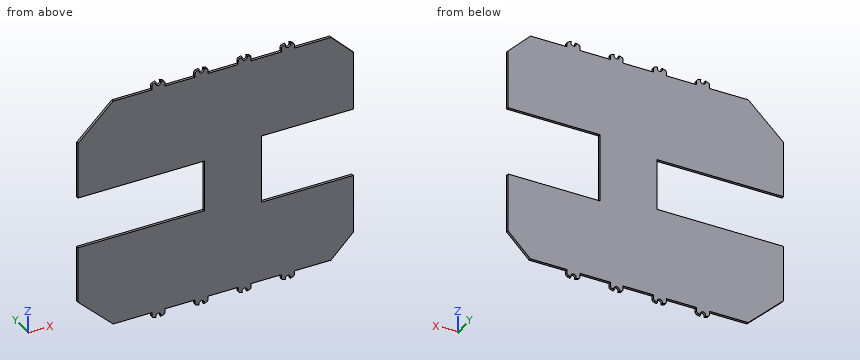
```python
from build123d import *

# Parameters (mm, degrees)
BOSS_EXTRUDE1_DEPTH  = 6
BOSS_EXTRUDE2_DEPTH  = 6
LPATTERN1_COUNT      = 4
LPATTERN1_PITCH      = 100
MIRROR1_COPY_1_DEPTH = 6
MIRROR1_COPY_2_DEPTH = 6
MIRROR1_COPY_3_DEPTH = 6


with BuildPart() as part:
    # Sketch1 → Boss-Extrude1 (new body)
    with BuildSketch(Plane(origin=(0, 0, 0), x_dir=(1, 0, 0), z_dir=(0, 1, 0))):
        Polygon((0, 160), (213, 160), (213, 297.159379566), (161.159379566, 349), (76.159379566, 349), (46.159379566, 349), (-343.622469374, 349), (-425, 271.691345905), (-425, 140), (-132, 140), (-132, 20), (-425, 20), (-425, -111.691345905), (-343.622469374, -189), (161.159379566, -189), (213, -137.159379566), (213, 0), (0, 0), align=None)
    extrude(amount=BOSS_EXTRUDE1_DEPTH)

    # Sketch1<3> → Boss-Extrude2 (add)
    with BuildSketch(Plane(origin=(0, 0, 0), x_dir=(1, 0, 0), z_dir=(0, 1, 0))):
        with BuildLine():
            Line((46.159379566, 349), (76.159379566, 349))
            Line((76.159379566, 349), (76.159379566, 357.347672364))
            ThreePointArc((76.159379566, 357.347672364), (75.196919236, 360.296955907), (72.680070199, 362.110812085))
            Line((72.680070199, 362.110812085), (66.259379566, 364.160696126))
            ThreePointArc((66.259379566, 364.160696126), (66.929994785, 362.643167673), (67.159379566, 361))
            ThreePointArc((67.159379566, 361), (59.516211894, 355.229384781), (56.059379566, 364.160696126))
            Line((56.059379566, 364.160696126), (49.638688934, 362.110812085))
            ThreePointArc((49.638688934, 362.110812085), (47.121839897, 360.296955907), (46.159379566, 357.347672364))
            Line((46.159379566, 357.347672364), (46.159379566, 349))
        make_face()
    boss_extrude2 = extrude(amount=BOSS_EXTRUDE2_DEPTH)

    # LPattern1: Boss-Extrude2 ×4
    with Locations(*[(-i * LPATTERN1_PITCH, 0, 0) for i in range(1, LPATTERN1_COUNT)]):
        add(boss_extrude2)

    # Mirror1: Boss-Extrude2 across plane
    add(boss_extrude2.mirror(Plane.XY.offset(-80)))

    # Mirror1 copy 1 sketch → Mirror1 copy 1 (add)
    with BuildSketch(Plane(origin=(-100, 0, -160), x_dir=(1, 0, 0), z_dir=(0, 1, 0))):
        with BuildLine():
            Line((46.159379566, -349), (76.159379566, -349))
            Line((76.159379566, -349), (76.159379566, -357.347672364))
            ThreePointArc((76.159379566, -357.347672364), (75.196919236, -360.296955907), (72.680070199, -362.110812085))
            Line((72.680070199, -362.110812085), (66.259379566, -364.160696126))
            ThreePointArc((66.259379566, -364.160696126), (66.929994785, -362.643167673), (67.159379566, -361))
            ThreePointArc((67.159379566, -361), (59.516211894, -355.229384781), (56.059379566, -364.160696126))
            Line((56.059379566, -364.160696126), (49.638688934, -362.110812085))
            ThreePointArc((49.638688934, -362.110812085), (47.121839897, -360.296955907), (46.159379566, -357.347672364))
            Line((46.159379566, -357.347672364), (46.159379566, -349))
        make_face()
    extrude(amount=MIRROR1_COPY_1_DEPTH)

    # Mirror1 copy 2 sketch → Mirror1 copy 2 (add)
    with BuildSketch(Plane(origin=(-200, 0, -160), x_dir=(1, 0, 0), z_dir=(0, 1, 0))):
        with BuildLine():
            Line((46.159379566, -349), (76.159379566, -349))
            Line((76.159379566, -349), (76.159379566, -357.347672364))
            ThreePointArc((76.159379566, -357.347672364), (75.196919236, -360.296955907), (72.680070199, -362.110812085))
            Line((72.680070199, -362.110812085), (66.259379566, -364.160696126))
            ThreePointArc((66.259379566, -364.160696126), (66.929994785, -362.643167673), (67.159379566, -361))
            ThreePointArc((67.159379566, -361), (59.516211894, -355.229384781), (56.059379566, -364.160696126))
            Line((56.059379566, -364.160696126), (49.638688934, -362.110812085))
            ThreePointArc((49.638688934, -362.110812085), (47.121839897, -360.296955907), (46.159379566, -357.347672364))
            Line((46.159379566, -357.347672364), (46.159379566, -349))
        make_face()
    extrude(amount=MIRROR1_COPY_2_DEPTH)

    # Mirror1 copy 3 sketch → Mirror1 copy 3 (add)
    with BuildSketch(Plane(origin=(-300, 0, -160), x_dir=(1, 0, 0), z_dir=(0, 1, 0))):
        with BuildLine():
            Line((46.159379566, -349), (76.159379566, -349))
            Line((76.159379566, -349), (76.159379566, -357.347672364))
            ThreePointArc((76.159379566, -357.347672364), (75.196919236, -360.296955907), (72.680070199, -362.110812085))
            Line((72.680070199, -362.110812085), (66.259379566, -364.160696126))
            ThreePointArc((66.259379566, -364.160696126), (66.929994785, -362.643167673), (67.159379566, -361))
            ThreePointArc((67.159379566, -361), (59.516211894, -355.229384781), (56.059379566, -364.160696126))
            Line((56.059379566, -364.160696126), (49.638688934, -362.110812085))
            ThreePointArc((49.638688934, -362.110812085), (47.121839897, -360.296955907), (46.159379566, -357.347672364))
            Line((46.159379566, -357.347672364), (46.159379566, -349))
        make_face()
    extrude(amount=MIRROR1_COPY_3_DEPTH)


solid = part.part
```
Model file for the job. Use its own axes, mm. Coordinates: 2 decimals unless noted, no trailing zeros. Loops run counter-clockwise (first coordinate to the right, second up) from the corner with the lowest first, then second, coordinate; pieces in that order, holes last. Notation, with made-up numbers: (58.5, 29.5) - (108.5, 29.5) arc R20 cw to (108.5, 53.5) - close; hole circle Ø8 at (61, 44). An arc over 180 degrees is marked (long way). Answer as a JSON object with one key per item and string values. Group by question number.
(1) Cut at A-A (x = -309). Give the cut face in (y, z), then the cut area to 3 significant figures.
(2) Cut at B-B (x = 105.5). Give the cut face in (y, z), then the cut area to 3 significant figures.
(3) Flat gauge pins, fed straight in: pin 1 (10 mm diameter, centred on x = 131.5, z = -205, fed in from -Y); pin 2 (1 mm diameter, centred on x = -118, y = 1, fed in from +Z); pin 3 (11 mm diameter, centred on x = -38.84, z = -361, fed in from +Y); pin 4 (3 mm diameter, centred on x = -100, y = 4.5, fed in from -Z). Where does each tip first touch, or does it go through?
(4) Cut at C-C (z = -79). Give the cut face in (x, y).
(5) Probe line 1 along Z through (x, y) = (-316.5, 4.7); line 2 along Z through (x, y) = (25.5, 3.35); line 3 along X through (y, z) = (4.3, -152). List the from-to ranges inside material, lowest first.
(6) Cut at D-D (z = 168). Give the cut face in (x, y), then the cut area to 3 significant figures.
Geometry says:
{
 "1": {"outline": "(0, -349) - (6, -349) - (6, -140) - (0, -140) - close; (0, -20) - (6, -20) - (6, 189) - (0, 189) - close", "area": "2,510 mm^2"},
 "2": {"outline": "(0, -349) - (6, -349) - (6, -160) - (0, -160) - close; (0, 0) - (6, 0) - (6, 189) - (0, 189) - close", "area": "2,270 mm^2"},
 "3": {"pin 1": "stops at y = 0", "pin 2": "stops at z = 189", "pin 3": "passes through", "pin 4": "stops at z = -349"},
 "4": {"outline": "(-132, 0) - (0, 0) - (0, 6) - (-132, 6) - close"},
 "5": {"line 1": "z = -349 to -140, -20 to 189", "line 2": "z = -349 to -160, 0 to 189", "line 3": "x = -425 to 0"},
 "6": {"outline": "(-365.73, 0) - (182.16, 0) - (182.16, 6) - (-365.73, 6) - close", "area": "3,290 mm^2"}
}
